For this review, take the finished solid that the model builds, in its own axes (mm). A direction names the side the tool comes from. Round coordinates to 2 decimals unless told otherwise and drop trailing zeros. Write each loop counter-clockwise with the first axis right and the second up, starting at its lowest first coordinate (ties: lowest second). Pieces come first, ordered by that corner, then holes. Notation, with made-up numbers: (67.25, 19.25) -> (97.25, 19.25) arc R24 cw to (97.25, 31.25) -> close; hole circle Ø6 at (32.25, 66). An arc over 180 degrees is marked (long way). Answer as CSV lines item,"result". Start each with the question number.
Item 1: Take a section at D-D on z = -17. Give the boundary of the cut face in (x, y), then the cut area to 3 significant figures.
Item 2: For pin 1 Ø4 at (x, z) = (93.417, 0) entering from -Y; pin 2 Ø3 at (x, y) = (-14, 6) entering from +Z; pin 3 Ø3.5 at (x, y) = (119.5, 2) entering from -Z; pin 4 Ø1 at (x, z) = (63, -40.5) entering from +Y, all flat-tipped, find the tip position at first contact; note any pin that passes through.
Item 3: Take a section at A-A on x = 125. Give the boundary of the cut face in (y, z).
Item 4: Machinability: for faces 1 (the cylindrical face through (60.01, 1.52, -0.51)), 2 (the cylindrical face through (-57.978, 5.028, 2.339)), which of the approach directions +Z, -Z, +X, -X, +Y, -Y give a long, thin tool a straight path to every point of the face, cutting with its end or side? Answer none if there is none.
Item 5: Take a section at B-B on x = 0. Give the boundary of the cut face in (y, z) (3 decimals), then the cut area to 3 significant figures.
Item 6: Wall thickness on probe 1 along Z at (x, y) = (125, 2.15); probe 2 along Z at (x, y) = (0, 2) (3 decimals); probe 3 along X at (y, z) = (2.25, -18): over which ranges is each line inside the solid? List them lowest first. Write a range as from..to.
Item 7: Take a section at C-C on z = 31. Give the boundary of the cut face in (x, y).
Item 8: Mouldability with a two-part tool opening along Z and no side actions: class faces 3 (the cylindrical face through (126.13, 1.52, 15.23)), 4 (the flat face through (59.132, 1.479, -40.023)), 5 (the cylindrical face through (-60.975, 3.549, 2.471)), 6 (the flat face through (54, 0, -1)) as +Z half, -Z half, draft (parallel to the pull), parting line (faces both ways), or undercut.
```python
from build123d import *

# Parameters (mm, degrees)
EXTRUDE_3_DEPTH     = 3
SKETCH_3_R          = 11.5
SKETCH_3_R_2        = 39
SKETCH_3_R_3        = 1.6
SKETCH_3_R_4        = 2.1
CUT_EXTRUDE_1_DEPTH = 4
SKETCH_4_W          = 3
SKETCH_4_H          = 4
SKETCH_6_W          = 30
SKETCH_6_H          = 10
CUT_EXTRUDE_3_DEPTH = 10


with BuildPart() as part:
    # 草图2 → 凸台-拉伸3 (new body)
    with BuildSketch(Plane(origin=(0, 0, 0), x_dir=(1, 0, 0), z_dir=(0, 1, 0))):
        with BuildLine():
            Line((91.901888805, 25), (25.431682676, 55.473238064))
            ThreePointArc((25.431682676, 55.473238064), (-61.025, 0), (25.431682676, -55.473238064))
            Line((25.431682676, -55.473238064), (91.901888805, -25))
            Line((91.901888805, -25), (130, -25))
            Line((130, -25), (130, 25))
            Line((130, 25), (91.901888805, 25))
        make_face()
    extrude(amount=EXTRUDE_3_DEPTH)

    # 草图3 → 切除-拉伸1 (cut, through all)
    with BuildSketch(Plane(origin=(0, 3, 0), x_dir=(1, 0, 0), z_dir=(0, 1, 0))):
        with Locations((71.5, 0)):
            Circle(SKETCH_3_R)
        Circle(SKETCH_3_R_2)
        with Locations((71.5, 21.917)):
            Circle(SKETCH_3_R_3)
        with Locations((93.417, 0)):
            Circle(SKETCH_3_R_3)
        with Locations((71.5, -21.917)):
            Circle(SKETCH_3_R_3)
        with Locations((125, 17)):
            Circle(SKETCH_3_R_4)
        with Locations((107, 17)):
            Circle(SKETCH_3_R_4)
        with Locations((125, -17)):
            Circle(SKETCH_3_R_4)
        with Locations((107, -17)):
            Circle(SKETCH_3_R_4)
    extrude(amount=-CUT_EXTRUDE_1_DEPTH, mode=Mode.SUBTRACT)

    # 草图4 → 旋转1 (revolve)
    with BuildSketch(Plane.XY):
        with Locations((-59.525, 5)):
            Rectangle(SKETCH_4_W, SKETCH_4_H)
    revolve(axis=Axis((0, 38.176517008, 0), (0, -1, 0)))

    # 草图6 → 切除-拉伸3 (cut)
    with BuildSketch(Plane(origin=(61.025, 0, 0), x_dir=(0, 0, -1), z_dir=(1, 0, 0))):
        with Locations((0, 8)):
            Rectangle(SKETCH_6_W, SKETCH_6_H)
    extrude(amount=-CUT_EXTRUDE_3_DEPTH, mode=Mode.SUBTRACT)


solid = part.part
```
Output values:
1,outline,"(-58.61, 0) -> (-35.1, 0) -> (-35.1, 3) -> (-55.48, 3) -> (-55.48, 7) -> (-58.61, 7) -> close; (35.1, 0) -> (104.9, 0) -> (104.9, 3) -> (58.61, 3) -> (58.61, 7) -> (55.48, 7) -> (55.48, 3) -> (35.1, 3) -> close; (109.1, 0) -> (122.9, 0) -> (122.9, 3) -> (109.1, 3) -> close; (127.1, 0) -> (130, 0) -> (130, 3) -> (127.1, 3) -> close"
1,area,"355 mm^2"
2,pin 1,"stops at y = 0"
2,pin 2,"stops at z = 59.73"
2,pin 3,"stops at z = -25"
2,pin 4,"passes through"
3,outline,"(0, -25) -> (3, -25) -> (3, -19.1) -> (0, -19.1) -> close; (0, -14.9) -> (3, -14.9) -> (3, 14.9) -> (0, 14.9) -> close; (0, 19.1) -> (3, 19.1) -> (3, 25) -> (0, 25) -> close"
4,face 1,"+Y, -Y"
4,face 2,"+Y"
5,outline,"(0, -61.025) -> (7, -61.025) -> (7, -58.025) -> (3, -58.025) -> (3, -39) -> (0, -39) -> close; (0, 39) -> (3, 39) -> (3, 58.025) -> (7, 58.025) -> (7, 61.025) -> (0, 61.025) -> close"
5,area,"156 mm^2"
6,probe 1,"z = -25..-19.1, -14.9..14.9, 19.1..25"
6,probe 2,"z = -61.025..-39, 39..61.025"
6,probe 3,"x = -58.31..-34.6, 34.6..105.15, 108.85..123.15, 126.85..130"
7,outline,"(-52.56, 0) -> (-23.66, 0) -> (-23.66, 3) -> (-49.05, 3) -> (-49.05, 7) -> (-52.56, 7) -> close; (23.66, 0) -> (78.81, 0) -> (78.81, 3) -> (52.56, 3) -> (52.56, 7) -> (49.05, 7) -> (49.05, 3) -> (23.66, 3) -> close"
8,face 3,"undercut"
8,face 4,"-Z half"
8,face 5,"parting line"
8,face 6,"draft"
